Source: CAD feature listing. Evaluate the final solid. Frame: model axes, mm. A direction names the side the tool comes from. Give positions to 0.01 mm unless a question says otherwise; leave off trailing zeros. Order: outer loops, then holes, each group sorted by start corner. A loop starts at its lowest first (then second) coordinate and runs counter-clockwise, first axis right, second up. Notation, with made-up numbers: (83.5, 35) -> (125.5, 35) arc R30 cw to (125.5, 74) -> close; hole circle Ø6 at (2.5, 70.5). An arc over 180 degrees is marked (long way). Answer in a Markdown table with one row per item.
Autodesk Fusion 360 part; units mm, degrees
sketch "Sketch1" plane through (0, 0, 0) normal (0, 1, 0) x (1, 0, 0)
  circle A0 centre (0, 0) radius 2.5
  circle A1 centre (0, 0) radius 4
  dimension "d1" = 5
  dimension "d2" = 8
extrude "Extrude1" add sketch "Sketch1" along normal blind 7.4
sketch "Sketch2" plane through (0, 7.4, 0) normal (0, 1, 0) x (-1, 0, 0)
  circle A0 centre (0, 0) radius 2.5
  circle A1 centre (0, 0) radius 4
  circle A2 centre (0, 0) radius 3
  dimension "d5" = 6
extrude "Extrude2" add sketch "Sketch2" along normal blind 4 contours A2
fillet "Fillet1" radius 1 1 edges at (-3.7293, 7.4, 1.4465)
(1) First-contact query: pin 1 Ø4 at (y, z) = (2, -0.5) entering from -X. Flat tip, straight axial feed; report the tip coordinate or a pass-through.
A:
| item | result |
|---|---|
| pin 1 | stops at x = -4 |
(2) Section query C-C (y = 1). Return the cut outline in (x, z), plus the area to 3 significant figures.
A:
| item | result |
|---|---|
| outline | circle Ø8 at (0, 0); hole circle Ø5 at (0, 0) |
| area | 30.6 mm^2 |
(3) Access query for faces 1 (the cylindrical face through (-0.867, 3.155, -3.905)), 2 (the cylindrical face through (3, 9, 0)). Directions: +Z, -Z, +X, -X, +Y, -Y. A direction counts if a zero-diameter tool reaches every point of the face in a straight line with its end or side. Return the directions, or none.
A:
| item | result |
|---|---|
| face 1 | +Y, -Y |
| face 2 | +Y |
(4) Section query B-B (y = 9.5). Return the cut outline in (x, z).
A:
| item | result |
|---|---|
| outline | circle Ø6 at (0, 0); hole circle Ø5 at (0, 0) |
(5) Ray query, probe 1 along Z at (x, y) = (0, 5.75); probe 2 along Z at (x, y) = (0, 8). Return the intervals inside material, ascending.
A:
| item | result |
|---|---|
| probe 1 | z = -4 to -2.5, 2.5 to 4 |
| probe 2 | z = -3 to -2.5, 2.5 to 3 |
